Design review of the part built by this model. Coordinates are the model's own, in mm. Face numbers are marked on the shaded views. A direction names the side the tool comes from. Give positions to 0.01 mm unless a question says otherwise; leave off trailing zeros. Order: outer loops, then holes, each group sorted by start corner. A loop starts at its lowest first (then second) coordinate and runs counter-clockwise, first axis right, second up.
Autodesk Inventor part; units mm, degrees
ref_plane "YZ Plane" through (0, 0, 0) normal (1, 0, 0) x (0, 1, 0)
ref_plane "XZ Plane" through (0, 0, 0) normal (0, 1, 0) x (-1, 0, 0)
ref_plane "XY Plane" through (0, 0, 0) normal (0, 0, 1) x (1, 0, 0)
sketch "Sketch1" plane through (0, 0, 0) normal (0, 1, 0) x (-1, 0, 0)
  line L0 (0, 0) -> (7, 0)
  line L1 (7, 0) -> (7, -10)
  line L2 (7, -10) -> (0, -10)
  line L3 (0, -10) -> (0, 0)
  line L4 (36.5, -60.1) -> (44.5, -60.1)
  line L5 (44.5, -60.1) -> (44.5, -53.1)
  line L6 (44.5, -53.1) -> (36.5, -53.1)
  line L7 (36.5, -53.1) -> (36.5, -60.1)
  line L8 (36.5, -53.1) -> (7, -10)
  line L9 (30.7235, -57.0537) -> (0.8012, -13.3368)
  line L10 (0.8012, -13.3368) -> (0, -12.1913)
  line L11 (0, -12.1913) -> (0, -10)
  line L12 (30.7235, -57.0537) -> (32.8378, -60.1)
  line L13 (32.8378, -60.1) -> (36.5, -60.1)
  dimension "d0" = 10
  dimension "d1" = 7
  dimension "d7" = 29.5
  dimension "d14" = 50.1
  dimension "d15" = 7
  dimension "d16" = 8
  dimension "d17" = 7
extrude "Extrusion1" add sketch "Sketch1" along normal blind 10
chamfer "Chamfer1" distance 2 angle 45 4 edges at (-44.5, 0, -56.6) (-44.5, 10, -56.6) (-3.5, 10, 0) (-3.5, 0, 0)
sketch "Sketch2" plane through (0, 0, -12.1913) normal (1, 0, 0) x (0, 0, -1)
  line L0 (-12.1913, 0) -> (-2.1913, 0) construction
  line L1 (-2.1913, 0) -> (-2.1913, 10) construction
  line L2 (-2.1913, 10) -> (-12.1913, 10) construction
  line L3 (-12.1913, 10) -> (-12.1913, 0) construction
  line L4 (-2.1913, 10) -> (-12.1913, 0) construction
  circle A0 centre (-7.1913, 5) radius 1.6
  dimension "d21" = 10
  dimension "d22" = 10
  dimension "d23" = 3.2
extrude "Extrusion2" cut sketch "Sketch2" against normal through all
sketch "Sketch3" plane through (-36.5, 0, -53.1) normal (0, 0, 1) x (1, 0, 0)
  line L0 (0, 0) -> (0, 10)
  line L1 (0, 10) -> (-10, 0) construction
  line L2 (0, 10) -> (14.1421, 10) construction
  line L3 (0, 5) -> (-3.5, 5)
  circle A0 centre (-3.5, 5) radius 1.5
  point P0 (36.5, 0)
  dimension "d26" = 135
  dimension "d27" = 3.5
  dimension "d28" = 3
extrude "Extrusion3" cut sketch "Sketch3" against normal blind 10
sketch "Sketch4" plane through (0, 0, -12.1913) normal (1, 0, 0) x (0, 0, -1)
  circle A0 centre (-7.1913, 5) radius 1.6
  circle A1 centre (-7.1913, 5) radius 3
  point P0 (-12.1913, 0)
  dimension "d31" = 6
extrude "Extrusion4" cut sketch "Sketch4" against normal blind 3.5
sketch "Sketch5" plane through (-36.5, 0, -53.1) normal (0, 0, 1) x (1, 0, 0)
  circle A0 centre (-3.5, 5) radius 3
  point P0 (36.5, 0)
  dimension "d34" = 6
extrude "Extrusion5" cut sketch "Sketch5" against normal blind 3.5
sketch "Sketch6" plane through (0, 10, 0) normal (0, 1, 0) x (1, 0, 0)
  line L0 (-7, 10) -> (-7, 2)
  line L1 (-7, 10) -> (-12, 10)
  line L2 (-12, 10) -> (-12, 17.3051)
  line L3 (-36.5, 53.1) -> (-7, 10)
  point P0 (0, 0)
  dimension "d37" = 5
  dimension "d38" = 90
extrude "Extrusion6" add sketch "Sketch6" against normal blind 10
sketch "Sketch7" plane through (0, 10, 0) normal (0, 1, 0) x (1, 0, 0)
  line L0 (-30.7235, 57.0537) -> (-32.8378, 60.1)
  line L1 (-32.8378, 60.1) -> (-36.4998, 60.1)
  line L2 (-32.8378, 60.1) -> (-42.5, 60.1)
  line L3 (-36.4998, 60.1) -> (-36.4998, 63.1)
  line L4 (-36.4998, 63.1) -> (-32.8378, 60.1)
  point P0 (0, 0)
  dimension "d41" = 3.662
  dimension "d42" = 3
extrude "Extrusion7" add sketch "Sketch7" against normal blind 10
properties part number "HoldingArms"
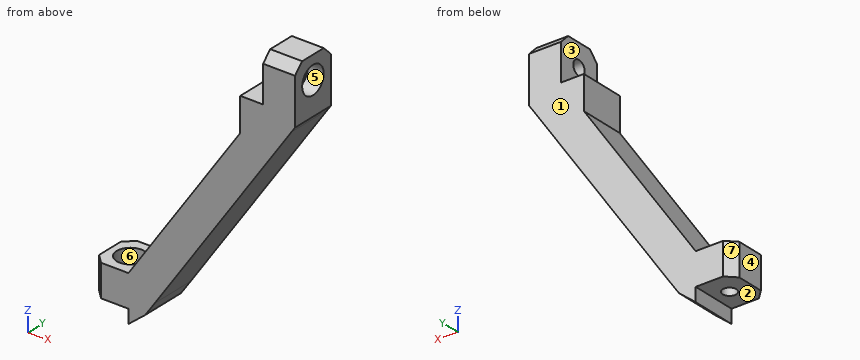
1. Take a section at D-D (y = 9). State the section outline as (x, z) points, then the cut area to 3 significant figures.
Recorded:
outline: (-43.5, -60.1) - (-36.5, -60.1) - (-36.5, -63.1) - (-32.84, -60.1) - (-30.72, -57.05) - (-0.8, -13.34) - (0, -12.19) - (0, -1) - (-7, -1) - (-7, -10) - (-12, -10) - (-12, -17.31) - (-36.5, -53.1) - (-43.5, -53.1) - close
area: 542 mm2
2. Draft analysis for pull direction Y (two halves, no side actions). For the marked faces 4, 5, 6 and 7, state which applies: pulls with the +Y half, pulls with the -Y half, needs draft (parallel to the pull), parting line crosses it, or undercut.
Recorded:
face 4: needs draft
face 5: undercut
face 6: undercut
face 7: pulls with the +Y half
3. Machinability: for the marked faces 1, 2 and 3, which of the approach directions +Z, -Z, +X, -X, +Y, -Y give a long, thin tool a straight path to every point of the face, cutting with its end or side? Answer none if there is none.
Recorded:
face 1: +Z, -Z, +X, -X, +Y
face 2: -Z, -X, +Y, -Y
face 3: +Z, -X, +Y, -Y
4. Take a section at A-A (x = -40). State the section outline as (y, z) points.
Recorded:
outline: (0, -60.1) - (3.5, -60.1) - (3.5, -56.6) - (2, -56.6) - (2, -53.1) - (0, -53.1) - close; (6.5, -60.1) - (10, -60.1) - (10, -53.1) - (8, -53.1) - (8, -56.6) - (6.5, -56.6) - close
5. Take a section at B-B (z = -5). State the section outline as (x, y) points.
Recorded:
outline: (-7, 0) - (0, 0) - (0, 2) - (-3.5, 2) - (-3.5, 3.4) - (-7, 3.4) - close; (-7, 6.6) - (-3.5, 6.6) - (-3.5, 8) - (0, 8) - (0, 10) - (-7, 10) - close
6. Take a section at C-C (y = 5). State how many separate pieces and enclosed holes the cut face has, then the cut area to 3 significant figures.
Recorded:
separate pieces: 3
enclosed holes: 0
area: 493 mm2
7. For pin 1 (5.5 mm diameter, centred on y = 5, z = -5, fed in from +X); pin 2 (3 mm diameter, centred on y = 5.5, z = -5.5, fed in from -X); pin 3 (4 mm diameter, centred on x = -7.5, y = 6.5, fed in from -Z), all flat-tipped, find the tip position at first contact; note any pin that passes through.
Recorded:
pin 1: stops at x = -3.5
pin 2: stops at x = -7
pin 3: stops at z = -26.05
8. For line 1 along Y through (x, z) = (-6.15, -5); line 2 along Y through (x, z) = (-1, -5); line 3 along Z through (x, y) = (-37.5, 4.75), list the stretches that pass through material, from the lowest coordinate up.
Recorded:
line 1: y = 0 to 3.4, 6.6 to 10
line 2: y = 0 to 2, 8 to 10
line 3: z = -60.1 to -56.6
